from build123d import *

# Parameters (mm, degrees)
ESQUISSE1_R      = 4
EXTRUSION1_DEPTH = 3
CONG_2_R         = 10
EXTRUSION2_REACH = 5
ESQUISSE3_R      = 2.5
EXTRUSION3_REACH = 5


with BuildPart() as part:
    # Esquisse1 → Extrusion1 (new body)
    with BuildSketch(Plane(origin=(0, 0, 0), x_dir=(1, 0, 0), z_dir=(0, 1, 0))):
        Polygon((-150, -105), (150, -105), (150, 0), (150, 85), (120, 115), (-120, 115), (-150, 85), (-150, 0), align=None)
        with Locations((0, 41.75)):
            Circle(ESQUISSE1_R, mode=Mode.SUBTRACT)
        with Locations((-96, 41.75)):
            Circle(ESQUISSE1_R, mode=Mode.SUBTRACT)
        with Locations((0, -41.75)):
            Circle(ESQUISSE1_R, mode=Mode.SUBTRACT)
        with Locations((-96, -41.75)):
            Circle(ESQUISSE1_R, mode=Mode.SUBTRACT)
        with Locations((96, -41.75)):
            Circle(ESQUISSE1_R, mode=Mode.SUBTRACT)
        with Locations((96, 41.75)):
            Circle(ESQUISSE1_R, mode=Mode.SUBTRACT)
        Polygon((-142.5, 55), (-142.5, -55), (-111.5, -55), (-111.5, -35.5), (-80.5, -35.5), (-80.5, 35.5), (-111.5, 35.5), (-111.5, 55), align=None, mode=Mode.SUBTRACT)
        Polygon((111.5, 55), (142.5, 55), (142.5, -55), (111.5, -55), (111.5, -35.5), (80.5, -35.5), (80.5, 35.5), (111.5, 35.5), align=None, mode=Mode.SUBTRACT)
    extrude(amount=EXTRUSION1_DEPTH)

    # Congé2
    cong_2_edges = [part.edges().sort_by_distance(p)[0] for p in [
        (150, 1.5, -85),
        (150, 1.5, 105),
        (-150, 1.5, 105),
        (-150, 1.5, -85),
        (-120, 1.5, -115),
        (120, 1.5, -115),
    ]]
    fillet(cong_2_edges, radius=CONG_2_R)

    # Esquisse3 → Extrusion2 (cut, up to next)
    with BuildSketch(Plane(origin=(0, 3, 0), x_dir=(1, 0, 0), z_dir=(0, 1, 0)), mode=Mode.PRIVATE) as extrusion2_sk1:
        with Locations((-140, -95)):
            Circle(ESQUISSE3_R)
    extrusion2_tool1 = extrude(extrusion2_sk1.sketch, amount=-EXTRUSION2_REACH, mode=Mode.PRIVATE) & part.part
    add(extrusion2_tool1.solids().sort_by_distance((-140, 3, 95))[0], mode=Mode.SUBTRACT)
    # Esquisse3 → Extrusion2 (cut, up to next)
    with BuildSketch(Plane(origin=(0, 3, 0), x_dir=(1, 0, 0), z_dir=(0, 1, 0)), mode=Mode.PRIVATE) as extrusion2_sk2:
        with Locations((-140, 80.857864376)):
            Circle(ESQUISSE3_R)
    extrusion2_tool2 = extrude(extrusion2_sk2.sketch, amount=-EXTRUSION2_REACH, mode=Mode.PRIVATE) & part.part
    add(extrusion2_tool2.solids().sort_by_distance((-140, 3, -80.857864))[0], mode=Mode.SUBTRACT)
    # Esquisse3 → Extrusion2 (cut, up to next)
    with BuildSketch(Plane(origin=(0, 3, 0), x_dir=(1, 0, 0), z_dir=(0, 1, 0)), mode=Mode.PRIVATE) as extrusion2_sk3:
        with Locations((-115.857864376, 105)):
            Circle(ESQUISSE3_R)
    extrusion2_tool3 = extrude(extrusion2_sk3.sketch, amount=-EXTRUSION2_REACH, mode=Mode.PRIVATE) & part.part
    add(extrusion2_tool3.solids().sort_by_distance((-115.857864, 3, -105))[0], mode=Mode.SUBTRACT)
    # Esquisse3 → Extrusion2 (cut, up to next)
    with BuildSketch(Plane(origin=(0, 3, 0), x_dir=(1, 0, 0), z_dir=(0, 1, 0)), mode=Mode.PRIVATE) as extrusion2_sk4:
        with Locations((140, -95)):
            Circle(ESQUISSE3_R)
    extrusion2_tool4 = extrude(extrusion2_sk4.sketch, amount=-EXTRUSION2_REACH, mode=Mode.PRIVATE) & part.part
    add(extrusion2_tool4.solids().sort_by_distance((140, 3, 95))[0], mode=Mode.SUBTRACT)
    # Esquisse3 → Extrusion2 (cut, up to next)
    with BuildSketch(Plane(origin=(0, 3, 0), x_dir=(1, 0, 0), z_dir=(0, 1, 0)), mode=Mode.PRIVATE) as extrusion2_sk5:
        with Locations((140, 80.857864376)):
            Circle(ESQUISSE3_R)
    extrusion2_tool5 = extrude(extrusion2_sk5.sketch, amount=-EXTRUSION2_REACH, mode=Mode.PRIVATE) & part.part
    add(extrusion2_tool5.solids().sort_by_distance((140, 3, -80.857864))[0], mode=Mode.SUBTRACT)
    # Esquisse3 → Extrusion2 (cut, up to next)
    with BuildSketch(Plane(origin=(0, 3, 0), x_dir=(1, 0, 0), z_dir=(0, 1, 0)), mode=Mode.PRIVATE) as extrusion2_sk6:
        with Locations((115.857864376, 105)):
            Circle(ESQUISSE3_R)
    extrusion2_tool6 = extrude(extrusion2_sk6.sketch, amount=-EXTRUSION2_REACH, mode=Mode.PRIVATE) & part.part
    add(extrusion2_tool6.solids().sort_by_distance((115.857864, 3, -105))[0], mode=Mode.SUBTRACT)

    # Esquisse4 → Extrusion3 (cut, up to next)
    with BuildSketch(Plane(origin=(0, 3, 0), x_dir=(1, 0, 0), z_dir=(0, 1, 0)), mode=Mode.PRIVATE) as extrusion3_sk1:
        Polygon((-90, -105), (-70, -85), (70, -85), (90, -105), align=None)
    extrusion3_tool1 = extrude(extrusion3_sk1.sketch, amount=-EXTRUSION3_REACH, mode=Mode.PRIVATE) & part.part
    add(extrusion3_tool1.solids().sort_by_distance((0, 3, 95.416667))[0], mode=Mode.SUBTRACT)


solid = part.part
Geometry: final body of the model. Coordinates: model frame, mm. A direction names the side the tool comes from. Coordinates: 2 decimals unless noted, no trailing zeros. Loops run counter-clockwise (first coordinate to the right, second up) from the corner with the lowest first, then second, coordinate; pieces in that order, holes last. Notation, with made-up numbers: (32, 16) - (75, 16) arc R13 cw to (75, 27) - close; hole circle Ø10 at (41.5, 13.5). An arc over 180 degrees is marked (long way). One line per question, with ' | ' between items. Start each with the question number.
(1) Cut plane C-C on x = 0. Output: boundary loops of the cut face in (y, z).
(2) Cut plane D-D on y = 1.4. Count the separate pieces of the cut face and the enclosed holes in it, and give its area (3 significant figures).
(3) Reachability of faces 5 (the cylindrical face through (-98.95, 1.48, -44.45)), 6 (the flat face through (80, 2, 95)) from +Z, -Z, +X, -X, +Y, -Y: full face, straight path, thin tool, end or side. Return the list, or none.
(4) Draft query along X for faces 1 (the cylindrical face through (-0.521, 1.479, -45.716)), 2 (the flat face through (-2, 0, -7)), 3 (the flat face through (-80, 2, 95)), 4 (the cylindrical face through (146.99, 1.52, 102.15)). Return one class per face: +X half, -X half, draft (parallel to the pull), parting line (faces both ways), or undercut.
(5) Cut plane A-A on z = -41.75. Output: boundary loops of the cut face in (x, y), and give its area (3 significant figures).
(6) Cut plane B-B on x = -96. Output: boundary loops of the cut face in (y, z), and give its area (3 significant figures).
(7) First-contact query: pin 1 (1 mm diameter, centred on x = 87, y = 1, fed in from +Z); pin 2 (1.5 mm diameter, centred on x = 129.5, y = 1, fed in from -Z). Flat tips, straight axial feed; report the tip coordinate or a pass-through.
(8) Ray query, L1, parallel to Z at x = -96, y = 0.6; L2, parallel to X at y = 2.4, z = -54; L3, parallel to X at y = 0.7, z = 41.75. Return the intervals inside material, ascending. Write a range as from..to.
Here are the results:
1) outline: (0, -115) - (3, -115) - (3, -45.75) - (0, -45.75) - close; (0, -37.75) - (3, -37.75) - (3, 37.75) - (0, 37.75) - close; (0, 45.75) - (3, 45.75) - (3, 85) - (0, 85) - close
2) separate pieces: 1 | enclosed holes: 14 | area: 50,200 mm²
3) face 5: +Y, -Y | face 6: +Z, +Y, -Y
4) face 1: undercut | face 2: draft | face 3: undercut | face 4: +X half
5) outline: (-150, 0) - (-142.5, 0) - (-142.5, 3) - (-150, 3) - close; (-111.5, 0) - (-100, 0) - (-100, 3) - (-111.5, 3) - close; (-92, 0) - (-4, 0) - (-4, 3) - (-92, 3) - close; (4, 0) - (92, 0) - (92, 3) - (4, 3) - close; (100, 0) - (111.5, 0) - (111.5, 3) - (100, 3) - close; (142.5, 0) - (150, 0) - (150, 3) - (142.5, 3) - close | area: 642 mm²
6) outline: (0, -115) - (3, -115) - (3, -45.75) - (0, -45.75) - close; (0, -37.75) - (3, -37.75) - (3, -35.5) - (0, -35.5) - close; (0, 35.5) - (3, 35.5) - (3, 37.75) - (0, 37.75) - close; (0, 45.75) - (3, 45.75) - (3, 105) - (0, 105) - close | area: 399 mm²
7) pin 1: z = 102.5 | pin 2: z = -106.25
8) L1: -115..-45.75, -37.75..-35.5, 35.5..37.75, 45.75..105 | L2: -150..-142.5, -111.5..111.5, 142.5..150 | L3: -150..-142.5, -111.5..-100, -92..-4, 4..92, 100..111.5, 142.5..150
